Drawing for the job (mm, zero at the part's lowest x, y, z). A direction names the side the tool comes from. Round coordinates to 2 decimals unless told otherwise and drop trailing zeros. Loops run counter-clockwise (first coordinate to the right, second up) from the corner with the lowest first, then second, coordinate; pieces in that order, holes last. Notation, with made-up numbers: M -22,50 L 19,50 A16 ccw 19,70 Z; hole C -4,-22.75 d8. An arc over 180 degrees is marked long. Use a Markdown table: item, result. Add a question column.
Q1. Cut at D-D (z = 31). Give the cut face in (x, y), plus the area to 3 significant figures.
Q2. Tool access for the marked faces 4, 5 and 6: list every direction of +Z, -Z, +X, -X, +Y, -Y with a clear straight run to the whole face (end or side of a thin tool).
Q3. Pin check, flat tips, straight feed: pin 1 (2.5 mm diameter, centred on x = 25.5, y = 10, fed in from -Z); pin 2 (3 mm diameter, centred on x = 26, y = 1.5, fed in from -Z); pin 3 (3 mm diameter, centred on x = 27.5, z = 37.5, fed in from +Y); pin 4 (1.4 mm diameter, centred on y = 9.5, z = 35, fed in from +X). Stop position of each tip, or through.
Q4. Probe line 1 (Z direction, x = 4.5, y = 1.5); line 2 (Z direction, x = 27, y = 2.75); line 3 (X direction, y = 4.25, z = 26.5). List the from-to ranges inside material, lowest first. Write a range as from..to.
Q5. Cut at A-A (z = 35). Give the cut face in (x, y).
Q6. Mould opens along X. For the marked faces 1, 2 and 3 say: +X half, -X half, draft (parallel to the pull), parting line (faces both ways), or undercut.
Q7. Cut at B-B (y = 1). Give the cut face in (x, z).
Q8. Cut at C-C (y = 9). Give the cut face in (x, z), plus the area to 3 significant figures.
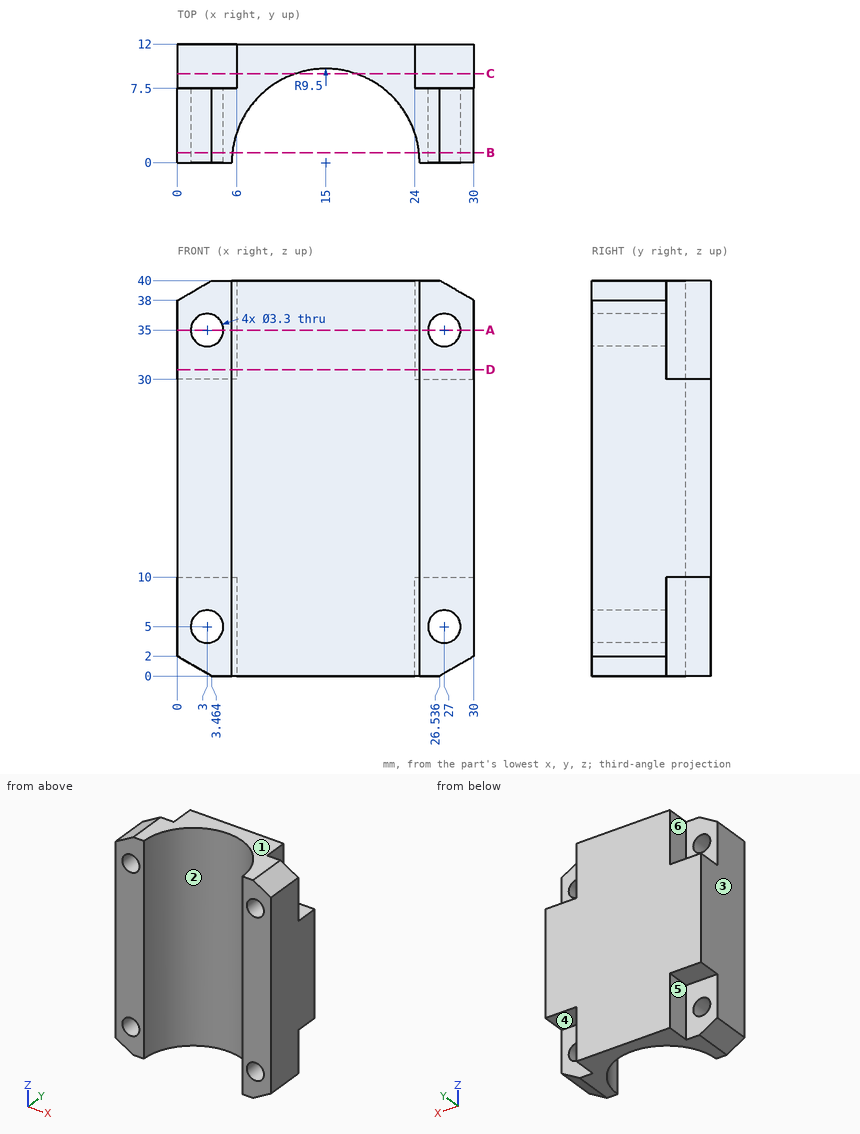
Checked values:
| question | item | result |
|---|---|---|
| 1 | outline | M 0,0 L 5.5,0 A9.5 cw 24.5,0 L 30,0 L 30,7.5 L 24,7.5 L 24,12 L 6,12 L 6,7.5 L 0,7.5 Z |
| 1 | area | 164 mm^2 |
| 2 | face 4 | -Z, +X, +Y |
| 2 | face 5 | -Z, -X, +Y |
| 2 | face 6 | +Z, -X, +Y |
| 3 | pin 1 | stops at z = 10 |
| 3 | pin 2 | stops at z = 0 |
| 3 | pin 3 | stops at y = 7.5 |
| 3 | pin 4 | stops at x = 24 |
| 4 | line 1 | z = 0..4.31, 5.69..34.31, 35.69..40 |
| 4 | line 2 | z = 0.27..3.35, 6.65..33.35, 36.65..39.73 |
| 4 | line 3 | x = 0..6.5, 23.5..30 |
| 5 | outline | M 0,0 L 1.35,0 L 1.35,7.5 L 0,7.5 Z; M 4.65,0 L 5.5,0 A9.5 cw 24.5,0 L 25.35,0 L 25.35,7.5 L 24,7.5 L 24,12 L 6,12 L 6,7.5 L 4.65,7.5 Z; M 28.65,0 L 30,0 L 30,7.5 L 28.65,7.5 Z |
| 6 | face 1 | draft |
| 6 | face 2 | undercut |
| 6 | face 3 | -X half |
| 7 | outline | M 0,2 L 3.46,0 L 5.55,0 L 5.55,40 L 3.46,40 L 0,38 Z; M 24.45,0 L 26.54,0 L 30,2 L 30,38 L 26.54,40 L 24.45,40 Z; hole C 3,5 d3.3; hole C 3,35 d3.3; hole C 27,5 d3.3; hole C 27,35 d3.3 |
| 8 | outline | M 0,10 L 6,10 L 6,0 L 11.96,0 L 11.96,40 L 6,40 L 6,30 L 0,30 Z; M 18.04,0 L 24,0 L 24,10 L 30,10 L 30,30 L 24,30 L 24,40 L 18.04,40 Z |
| 8 | area | 717 mm^2 |
